from build123d import *

# Parameters (mm, degrees)
SKETCH1_W           = 185
SKETCH1_H           = 185
SKETCH1_W_2         = 140
SKETCH1_H_2         = 13
BOSS_EXTRUDE1_DEPTH = 5
SKETCH2_W           = 140
SKETCH2_H           = 13
BOSS_EXTRUDE2_DEPTH = 30
SKETCH4_W           = 140
SKETCH4_H           = 7
BOSS_EXTRUDE3_DEPTH = 30
CUT_EXTRUDE1_DEPTH  = 1000
SKETCH6_W           = 115
SKETCH6_H           = 115
CUT_EXTRUDE2_DEPTH  = 1000
SKETCH7_R           = 2.25
CUT_EXTRUDE3_DEPTH  = 1000
FILLET1_R           = 15
FILLET2_R           = 5
FILLET3_R           = 10


with BuildPart() as part:
    # Sketch1 → Boss-Extrude1 (new body)
    with BuildSketch(Plane(origin=(0, 0, 0), x_dir=(1, 0, 0), z_dir=(0, 1, 0))):
        with Locations((9.076200418, 24.041155145)):
            Rectangle(SKETCH1_W, SKETCH1_H)
        with Locations((9.076200418, -74.958844855)):
            Rectangle(SKETCH1_W_2, SKETCH1_H_2)
        with Locations((9.076200418, 123.041155145)):
            Rectangle(SKETCH1_W_2, SKETCH1_H_2)
    extrude(amount=BOSS_EXTRUDE1_DEPTH)

    # Sketch2 → Boss-Extrude2 (add)
    with BuildSketch(Plane(origin=(0, 5, 0), x_dir=(1, 0, 0), z_dir=(0, 1, 0))):
        with Locations((9.076200418, 123.041155145)):
            Rectangle(SKETCH2_W, SKETCH2_H)
        with Locations((9.076200418, -74.958844855)):
            Rectangle(SKETCH2_W, SKETCH2_H)
    extrude(amount=BOSS_EXTRUDE2_DEPTH)

    # Sketch4 → Boss-Extrude3 (add)
    with BuildSketch(Plane(origin=(0, 35, 0), x_dir=(1, 0, 0), z_dir=(0, 1, 0))):
        with Locations((9.076200418, 120.041155145)):
            Rectangle(SKETCH4_W, SKETCH4_H)
        with Locations((9.076200418, -71.958844855)):
            Rectangle(SKETCH4_W, SKETCH4_H)
    extrude(amount=BOSS_EXTRUDE3_DEPTH)

    # Sketch5 → Cut-Extrude1 (cut)
    with BuildSketch(Plane.XY.offset(75.458844855)):
        with BuildLine():
            Line((-40.923799582, 57.25), (59.076200418, 57.25))
            ThreePointArc((59.076200418, 57.25), (61.326200418, 55), (59.076200418, 52.75))
            Line((59.076200418, 52.75), (-40.923799582, 52.75))
            ThreePointArc((-40.923799582, 52.75), (-43.173799582, 55), (-40.923799582, 57.25))
        make_face()
    extrude(amount=-CUT_EXTRUDE1_DEPTH, mode=Mode.SUBTRACT)

    # Sketch6 → Cut-Extrude2 (cut)
    with BuildSketch(Plane(origin=(0, 5, 0), x_dir=(1, 0, 0), z_dir=(0, 1, 0))):
        with Locations((9.076200418, 24.041155145)):
            Rectangle(SKETCH6_W, SKETCH6_H)
    extrude(amount=-CUT_EXTRUDE2_DEPTH, mode=Mode.SUBTRACT)

    # Sketch7 → Cut-Extrude3 (cut)
    with BuildSketch(Plane(origin=(0, 5, 0), x_dir=(1, 0, 0), z_dir=(0, 1, 0))):
        with Locations(Location((-60.923799582, 94.041155145, 0), (0, 0, 270))):
            Circle(SKETCH7_R)
        with Locations(Location((79.076200418, 94.041155145, 0), (0, 0, 270))):
            Circle(SKETCH7_R)
        with Locations(Location((79.076200418, -45.958844855, 0), (0, 0, 270))):
            Circle(SKETCH7_R)
        with Locations(Location((-60.923799582, -45.958844855, 0), (0, 0, 270))):
            Circle(SKETCH7_R)
    extrude(amount=-CUT_EXTRUDE3_DEPTH, mode=Mode.SUBTRACT)

    # Fillet1
    fillet1_edges = [part.edges().sort_by_distance(p)[0] for p in [
        (-48.423799582, 2.5, 33.458844855),
        (-48.423799582, 2.5, -81.541155145),
        (66.576200418, 2.5, -81.541155145),
        (66.576200418, 2.5, 33.458844855),
        (101.576200418, 2.5, 68.458844855),
        (-83.423799582, 2.5, 68.458844855),
        (-83.423799582, 2.5, -116.541155145),
        (101.576200418, 2.5, -116.541155145),
    ]]
    fillet(fillet1_edges, radius=FILLET1_R)

    # Fillet2
    fillet2_edges = [part.edges().sort_by_distance(p)[0] for p in [
        (79.076200418, 17.5, 81.458844855),
        (-60.923799582, 17.5, 81.458844855),
        (-60.923799582, 17.5, -129.541155145),
        (79.076200418, 17.5, -129.541155145),
    ]]
    fillet(fillet2_edges, radius=FILLET2_R)

    # Fillet3
    fillet3_edges = [part.edges().sort_by_distance(p)[0] for p in [
        (9.076200418, 5, -116.541155145),
        (9.076200418, 5, 68.458844855),
    ]]
    fillet(fillet3_edges, radius=FILLET3_R)


solid = part.part
Here's how the part is built. I have some questions about the finished solid (model axes, mm). A direction names the side the tool comes from. Give positions to 0.01 mm unless a question says otherwise; leave off trailing zeros. Write each loop counter-clockwise with the first axis right and the second up, starting at its lowest first coordinate (ties: lowest second). Pieces come first, ordered by that corner, then holes. Notation, with made-up numbers: (12, 72.5) -> (71, 72.5) arc R9 ccw to (71, 77.5) -> close; hole circle Ø11 at (52.5, -8). An arc over 180 degrees is marked (long way). Use one line per item in the form item = value. Start each with the question number.
1. On a 3-axis mill with a long thin cutter (end or side, diameter ignored), from which of +Z, -Z, +X, -X, +Y, -Y can I reach the whole of each face in a straight line? I mean faces 1 (the face through (8, 40, 68.459)), 2 (the face through (83, 2, -116.541)), 3 (the face through (8, 50, 75.459)), 4 (the face through (8, 57.25, 72)), 5 (the face through (66.576, 3, -23)). Say none if no direction works.
2. If I drill on L1, parallel to Z at x = 27, y = 32; L2, parallel to Z at x = -44, y = 47; L3, parallel to Y at x = 83.5, z = -72, over which ranges is the centre line in solid material (lowest first)?
3. Imagine slicing it at B-B on y = 25.5. List the corners of the cut face in (x, z) for me.
4. Imagine slicing it at A-A on z = -63. List the corners of the cut face in (x, y) for me, plus the area to 3 significant figures.
5. Will these pins go through, and if not, where does the flat tip stop? pin 1 Ø4 at (x, y) = (-66, 2.5) entering from -Z; pin 2 Ø14.5 at (y, z) = (47.5, -114) entering from +X; pin 3 Ø2.5 at (x, y) = (-63.5, 2.5) entering from +Z.
6. Imagine slicing it at C-C on y = 42.5. List the corners of the cut face in (x, z) for me, plus the area to 3 significant figures.
7. Thinking about a two-plate mould opening in Y: for faces 6 (the face through (62.3, 2.46, -77.03)), 7 (the face through (8, 5, 36)), 8 (the face through (61.326, 55.049, -119.992)), which applies, +Y half, -Y half, draft (parallel to the pull), parting line (faces both ways), or undercut?
8. Imagine slicing it at D-D on z = -110. List the corners of the cut face in (x, y) for me, plus the area to 3 significant figures.
Entries:
q1.face_1 = +X, -X, +Y
q1.face_2 = -Z, +X, +Y, -Y
q1.face_3 = +Z, +X, -X, +Y
q1.face_4 = +Z, -Z
q1.face_5 = +Y, -Y
q2.L1 = -129.54 to -116.54, 68.46 to 81.46
q2.L2 = -123.54 to -116.54, 68.46 to 75.46
q2.L3 = 0 to 5
q3.outline = (-60.92, -124.54) arc R5 ccw to (-55.92, -129.54) -> (74.08, -129.54) arc R5 ccw to (79.08, -124.54) -> (79.08, -116.54) -> (-60.92, -116.54) -> close; (-60.92, 68.46) -> (79.08, 68.46) -> (79.08, 76.46) arc R5 ccw to (74.08, 81.46) -> (-55.92, 81.46) arc R5 ccw to (-60.92, 76.46) -> close
q4.outline = (-83.42, 0) -> (-48.42, 0) -> (-48.42, 5) -> (-83.42, 5) -> close; (66.58, 0) -> (101.58, 0) -> (101.58, 5) -> (66.58, 5) -> close
q4.area = 350 mm²
q5.pin_1 = -116.54
q5.pin_2 = 79.08
q5.pin_3 = 68.46
q6.outline = (-60.92, -123.54) -> (79.08, -123.54) -> (79.08, -116.54) -> (-60.92, -116.54) -> close; (-60.92, 68.46) -> (79.08, 68.46) -> (79.08, 75.46) -> (-60.92, 75.46) -> close
q6.area = 1,960 mm²
q7.face_6 = draft
q7.face_7 = +Y half
q7.face_8 = undercut
q8.outline = (-80.81, 0) -> (98.96, 0) -> (98.96, 5) -> (79.08, 5) -> (79.08, 5.62) -> (-60.92, 5.62) -> (-60.92, 5) -> (-80.81, 5) -> close
q8.area = 985 mm²
